Model file for the job. Use its own axes, mm. A direction names the side the tool comes from. Coordinates: 2 decimals unless noted, no trailing zeros. Write each loop counter-clockwise with the first axis right and the second up, starting at its lowest first coordinate (ties: lowest second). Pieces come first, ordered by that corner, then holes. Notation, with made-up numbers: (13.5, -35.75) - (65.5, -35.75) arc R12 ccw to (65.5, -22.75) - close; hole circle Ø7 at (36.25, 23). An arc over 180 degrees is marked (long way). Put each result on its own line as item: value. Start each with the question number.
1. Saw through at C-C, the plane z = -11.5. Write the cut outline in (x, y).
2. Pull direction X, two halves, no side cores. Call faces 4 (the face through (-74.049, 14.565, -5.323)), 5 (the face through (-5.948, 11.586, -1.521)), 6 (the face through (-73, 34.845, -7)): released by +X, released by -X, zero draft, split by the parting line, or undercut.
3. Drill centre lines: L1, parallel to Y at x = -75, z = -6; L2, parallel to Y at x = -16.5, z = -1.5; L3, parallel to Z at x = -14.5, y = -1. Where is each one in solid material? Low to high. Write a range as from..to.
4. Saw through at B-B, the plane x = -67. Write the cut outline in (y, z).
5. Which spindle directions (+Z, -Z, +X, -X, +Y, -Y) get a long thin tool onto all of the face, cutting with end or side? Do faces 1 (the face through (-34, 4, -3)), 2 (the face through (-71.7, 4.9, -5.7)), 3 (the face through (-64.09, 24, -1.28)). Say none if no direction does.
6. Drop flat-ended pins along their axis: P1, Ø6, axis at y = 21.5, z = -6.5, coming from the -X side; P2, Ø3, axis at y = 26, z = -5.5, coming from the +X side; P3, Ø1.2, axis at x = -26.58, y = 10.59, coming from the +Z side (3 decimals); P4, Ø1.5, axis at x = -46, z = -1.5, coming from the +Y side (3 decimals). Give the stop position or say it passes through.
7. Saw through at A-A, the plane y = 2. Write the cut outline in (x, z), plus the area to 3 significant figures.
```python
from build123d import *

# Parameters (mm, degrees)
F0_W     = 25
F0_H     = 18
F0_W_2   = 36
F1_DEPTH = 3
F2_D     = 2
F2_DEPTH = 8
F2_TIP   = 0.600860619
F4_W     = 21
F4_H     = 18
F4_H_2   = 22
F5_DEPTH = 3
F6_D     = 3.4
F6_DEPTH = 8
F6_TIP   = 1.0214630523


with BuildPart() as f1:
    # F0 (on Top) → F1 (new body)
    with BuildSketch(Plane.XY):
        with Locations((-16.3281254843, 3.8449834271)):
            Rectangle(F0_W, F0_H)
        with Locations((-46.8281254843, 3.8449834271)):
            Rectangle(F0_W_2, F0_H)
    extrude(amount=-F1_DEPTH)

    # F2
    with Locations(Plane.XY):
        with Locations((-26.5781254843, 10.5949834271), (-6.0781254843, 10.5949834271), (-6.0781254843, -2.9050165729), (-26.5781254843, -2.9050165729)):
            Hole(F2_D / 2, depth=F2_DEPTH)
            with Locations((0, 0, -(F2_DEPTH + F2_TIP / 2))):  # 118° drill point
                Cone(0, F2_D / 2, F2_TIP, mode=Mode.SUBTRACT)

    # F4 (on line) → F5 (join)
    with BuildSketch(Plane(origin=(-16.2070313711, 0, 28.0714017746), x_dir=(0.8660254038, 0, 0.5), z_dir=(0.5, 0, -0.8660254038))):
        with Locations((-66.6428035491, -3.8449834271)):
            Rectangle(F4_W, F4_H)
        with Locations((-66.6428035491, -23.8449834271)):
            Rectangle(F4_W, F4_H_2)
    extrude(amount=F5_DEPTH)

    # F6
    with Locations(Plane(origin=(-16.2070313711, 0, 28.0714017746), x_dir=(0.8660254038, 0, 0.5), z_dir=(-0.5, 0, 0.8660254038))):
        with Locations((-66.6428035491, 24.8449834271), (-66.6428035491, 4.8449834271)):
            Hole(F6_D / 2, depth=F6_DEPTH)
            with Locations((0, 0, -(F6_DEPTH + F6_TIP / 2))):  # 118° drill point
                Cone(0, F6_D / 2, F6_TIP, mode=Mode.SUBTRACT)


solid = f1.part
```
Final values:
1. outline: (-82.44, -5.16) - (-78.75, -5.16) - (-78.75, 34.84) - (-82.44, 34.84) - close
2. face 4: released by -X
2. face 5: undercut
2. face 6: zero draft
3. L1: y = -5.16..3.76, 5.93..23.76, 25.93..34.84
3. L2: y = -5.16..12.84
3. L3: z = -3..0
4. outline: (-5.16, -4.72) - (34.84, -4.72) - (34.84, -1.25) - (-5.16, -1.25) - close
5. face 1: -Z, +X, +Y, -Y
5. face 2: none
5. face 3: +Z, +X, +Y
6. P1: stops at x = -81.28
6. P2: stops at x = -65.76
6. P3: passes through
6. P4: stops at y = 12.845
7. outline: (-83.01, -10.5) - (-81.51, -13.1) - (-64.02, -3) - (-3.83, -3) - (-3.83, 0) - (-64.83, 0) - close
7. area: 244 mm²
